from build123d import *

# Parameters (mm, degrees)
ESBO_O1_R                = 2.75
RESSALTO_EXTRUS_O1_DEPTH = 3
CORTE_EXTRUS_O1_DEPTH    = 1.5
FILETE1_R                = 0.25
FILETE2_R                = 0.1
ESBO_O3_R                = 1.5
RESSALTO_EXTRUS_O2_DEPTH = 8


with BuildPart() as part:
    # Esboço1 → Ressalto-extrusão1 (new body)
    with BuildSketch(Plane(origin=(0, 0, 0), x_dir=(1, 0, 0), z_dir=(0, 1, 0))):
        with Locations(Location((0, 0, 0), (0, 0, 270))):
            Circle(ESBO_O1_R)
    extrude(amount=RESSALTO_EXTRUS_O1_DEPTH)

    # Esboço2 → Corte-extrusão1 (cut)
    with BuildSketch(Plane(origin=(0, 3, 0), x_dir=(1, 0, 0), z_dir=(0, 1, 0))):
        Polygon((0, 1.443375673), (-1.25, 0.721687836), (-1.25, -0.721687836), (0, -1.443375673), (1.25, -0.721687836), (1.25, 0.721687836), align=None)
    extrude(amount=-CORTE_EXTRUS_O1_DEPTH, mode=Mode.SUBTRACT)

    # Filete1
    filete1_edges = [part.edges().sort_by_distance(p)[0] for p in [
        (0, 3, -2.75),
    ]]
    fillet(filete1_edges, radius=FILETE1_R)

    # Filete2
    filete2_edges = [part.edges().sort_by_distance(p)[0] for p in [
        (0, 0, -2.75),
    ]]
    fillet(filete2_edges, radius=FILETE2_R)

    # Esboço3 → Ressalto-extrusão2 (add)
    with BuildSketch(Plane.XZ):
        with Locations(Location((0, 0, 0), (0, 0, 90))):
            Circle(ESBO_O3_R)
    extrude(amount=RESSALTO_EXTRUS_O2_DEPTH)


solid = part.part
Geometry check sheet. Reference: the model listing, model coordinates, mm. A direction names the side the tool comes from. Coordinates: 2 decimals unless noted, no trailing zeros. Order: outer loops, then holes, each group sorted by start corner. A loop starts at its lowest first (then second) coordinate and runs counter-clockwise, first axis right, second up. Notation, with made-up numbers: (0, 6) -> (31, 6) arc R25 cw to (31, 35) -> close; hole circle Ø4 at (-11, 2.5). An arc over 180 degrees is marked (long way). Use a Markdown table: item, result. Add a question column.
1. Material ranges on L1, parallel to Y at x = 1.2, z = 0.5; L2, parallel to Y at x = -1.5, z = -1.75; L3, parallel to Z at x = 0.35, y = 1, recorded low to high.
2. Cross-section at A-A (z = 0). Enter the section's corners in (x, y), and give its area (3 significant figures).
3. Mould release check, pull along Z, two halves, no side actions. Record for faces 1 (the face through (-0.45, -3.94, 1.43)), 2 (the face through (-0.63, 2.26, 1.08)), 3 (the face through (0, -8, 0)): pulls with the +Z half, pulls with the -Z half, needs draft (parallel to the pull), parting line crosses it, or undercut.
4. Cross-section at C-C (y = 0.75). Enter the section's corners in (x, z).
5. Set-up check for faces 4 (the face through (0, 0, 2)), 5 (the face through (-1.1, 3, 1.1)), 6 (the face through (0, 1.5, 0)): record each of +Z, -Z, +X, -X, +Y, -Y from which the full face is reachable in a straight line by a thin tool's end or side.
6. Cross-section at B-B (y = -0.5). Enter the section's corners in (x, z), and give its area (3 significant figures).
Filled sheet:
| question | item | result |
|---|---|---|
| 1 | L1 | -8 to 1.5 |
| 1 | L2 | 0 to 3 |
| 1 | L3 | -2.73 to 2.73 |
| 2 | outline | (-2.75, 0.1) arc R0.1 ccw to (-2.65, 0) -> (-1.5, 0) -> (-1.5, -8) -> (1.5, -8) -> (1.5, 0) -> (2.65, 0) arc R0.1 ccw to (2.75, 0.1) -> (2.75, 2.75) arc R0.25 ccw to (2.5, 3) -> (1.25, 3) -> (1.25, 1.5) -> (-1.25, 1.5) -> (-1.25, 3) -> (-2.5, 3) arc R0.25 ccw to (-2.75, 2.75) -> close |
| 2 | area | 36.7 mm2 |
| 3 | face 1 | parting line crosses it |
| 3 | face 2 | undercut |
| 3 | face 3 | needs draft |
| 4 | outline | circle Ø5.5 at (0, 0) |
| 5 | face 4 | -Y |
| 5 | face 5 | +Z, -Z, +X, -X, +Y |
| 5 | face 6 | +Y |
| 6 | outline | circle Ø3 at (0, 0) |
| 6 | area | 7.07 mm2 |
